from build123d import *

# Parameters (mm, degrees)
F1_W      = 2334
F1_H      = 613
F2_DEPTH  = 30
F3_W      = 45
F3_H      = 420
F3_W_2    = 982.5
F3_H_2    = 45
F4_DEPTH  = 70
F5_DEPTH  = 870
F8_W      = 45
F8_H      = 420
F9_DEPTH  = 70
F10_DEPTH = 670
F11_DEPTH = 70


# Not quite as in the source:
# - a feature names something its author has since deleted; it is built from what else it names


with BuildPart() as f2:
    # F1 (on offset) → F2 (new body)
    with BuildSketch(Plane.XY.offset(900)):
        Rectangle(F1_W, F1_H)
    extrude(amount=-F2_DEPTH)

    # F3 (on face) → F4 (join)
    with BuildSketch(Plane(origin=(0, 0, 870), x_dir=(1, 0, 0), z_dir=(0, 0, -1))):
        with Locations((-1102.5, 0)):
            Rectangle(F3_W, F3_H)
        with Locations((1102.5, 0)):
            Rectangle(F3_W, F3_H)
        with Locations((-538.75, 232.5)):
            Rectangle(F3_W_2, F3_H_2)
        with Locations((-538.75, -232.5)):
            Rectangle(F3_W_2, F3_H_2)
        Polygon((47.5, 255), (-47.5, 255), (-47.5, 210), (-22.5, 210), (22.5, 210), (47.5, 210), align=None)
        with Locations((538.75, 232.5)):
            Rectangle(F3_W_2, F3_H_2)
        Polygon((22.5, 210), (-22.5, 210), (-22.5, -210), (22.5, -210), (22.5, -47.5), (22.5, 47.5), align=None)
        with Locations((538.75, -232.5)):
            Rectangle(F3_W_2, F3_H_2)
    extrude(amount=F4_DEPTH)

    # F3 (on face) → F5 (join)
    with BuildSketch(Plane(origin=(0, 0, 870), x_dir=(1, 0, 0), z_dir=(0, 0, -1))):
        Polygon((-1030, 255), (-1125, 255), (-1125, 210), (-1080, 210), (-1030, 210), align=None)
        Polygon((47.5, 255), (-47.5, 255), (-47.5, 210), (-22.5, 210), (22.5, 210), (47.5, 210), align=None)
        Polygon((-1080, -210), (-1125, -210), (-1125, -255), (-1030, -255), (-1030, -210), align=None)
        Polygon((1125, 255), (1030, 255), (1030, 210), (1080, 210), (1125, 210), align=None)
        Polygon((22.5, -210), (-22.5, -210), (-47.5, -210), (-47.5, -255), (47.5, -255), (47.5, -210), align=None)
        Polygon((1125, -255), (1125, -210), (1080, -210), (1030, -210), (1030, -255), align=None)
    extrude(amount=F5_DEPTH)

    # F8 (on offset) → F9 (join)
    with BuildSketch(Plane.XY.offset(130)):
        Polygon((-638, 210), (-638, 255), (-1100, 255), (-1100, -255), (-638, -255), (-638, -210), (-1055, -210), (-1055, 210), align=None)
        Polygon((568, 210), (568, 255), (-568, 255), (-568, 210), (-22.5, 210), (22.5, 210), align=None)
        Polygon((-568, -255), (568, -255), (568, -210), (22.5, -210), (-22.5, -210), (-568, -210), align=None)
        Rectangle(F8_W, F8_H)
        Polygon((1100, -255), (1100, 255), (638, 255), (638, 210), (1055, 210), (1055, -210), (638, -210), (638, -255), align=None)
    extrude(amount=F9_DEPTH)

    # F8 (on offset) → F10 (join, through all)
    with BuildSketch(Plane.XY.offset(130)):
        Polygon((-638, -255), (-568, -255), (-568, -210), (-580.5, -210), (-625.5, -210), (-638, -210), align=None)
        Polygon((-568, 210), (-568, 255), (-638, 255), (-638, 210), (-625.5, 210), (-580.5, 210), align=None)
        Polygon((638, 210), (638, 255), (568, 255), (568, 210), (580.5, 210), (625.5, 210), align=None)
        Polygon((568, -255), (638, -255), (638, -210), (625.5, -210), (580.5, -210), (568, -210), align=None)
    extrude(amount=F10_DEPTH)

    # F8 (on offset) → F11 (join)
    with BuildSketch(Plane.XY.offset(130)):
        with Locations((-603, 0)):
            Rectangle(F8_W, F8_H)
        with Locations((603, 0)):
            Rectangle(F8_W, F8_H)
    extrude(amount=F11_DEPTH)


solid = f2.part
Could you check a few things on this model? Use its own coordinates, in mm. A direction names the side the tool comes from. Coordinates: 2 decimals unless noted, no trailing zeros. Write each loop counter-clockwise with the first axis right and the second up, starting at its lowest first coordinate (ties: lowest second). Pieces come first, ordered by that corner, then holes. Notation, with made-up numbers: (-38, -37.75) - (-10, -37.75) arc R15 cw to (-10, -16.75) - close; hole circle Ø3 at (27, -19). An arc over 180 degrees is marked (long way). Write item = value, one per line.
1) Suppose I cut it at B-B on z = 99. Please give me the cut outline in (x, y).
Result set:
outline = (-1125, -255) - (-1030, -255) - (-1030, -210) - (-1125, -210) - close; (-1125, 210) - (-1030, 210) - (-1030, 255) - (-1125, 255) - close; (-47.5, -255) - (47.5, -255) - (47.5, -210) - (-47.5, -210) - close; (-47.5, 210) - (47.5, 210) - (47.5, 255) - (-47.5, 255) - close; (1030, -255) - (1125, -255) - (1125, -210) - (1030, -210) - close; (1030, 210) - (1125, 210) - (1125, 255) - (1030, 255) - close
2) Suppose I cut it at A-A on x = -153.5. Please give me the cut outline in (y, z).
Result set:
outline = (-306.5, 870) - (-255, 870) - (-255, 800) - (-210, 800) - (-210, 870) - (210, 870) - (210, 800) - (255, 800) - (255, 870) - (306.5, 870) - (306.5, 900) - (-306.5, 900) - close; (-255, 130) - (-210, 130) - (-210, 200) - (-255, 200) - close; (210, 130) - (255, 130) - (255, 200) - (210, 200) - close
3) We'd pull the mould along Y, two halves only. Please class faces 1 (the flat face through (304, 232, 800)), 2 (the flat face through (580.5, -3, 165)): +Y half, -Y half, draft (parallel to the pull), parting line (faces both ways), or undercut.
Result set:
face_1 = draft
face_2 = undercut
4) Will these pins go through, and if not, where does the flat tip stop? pin 1 Ø3 at (x, y) = (652.5, -45.5) entering from -Z; pin 2 Ø21 at (y, z) = (55.5, 181.5) entering from -X; pin 3 Ø1 at (x, y) = (587.5, -33) entering from -Z.
Result set:
pin_1 = 870
pin_2 = -1100
pin_3 = 130
5) Please list where these lines run through material, in increasing order: line 1 (X direction, y = 246, z = 449); line 2 (X direction, y = 101, z = 192.5); line 3 (Y direction, x = 158.5, z = 173.5). Write a range as [from, to].
Result set:
line_1 = [-1125, -1030], [-638, -568], [-47.5, 47.5], [568, 638], [1030, 1125]
line_2 = [-1100, -1055], [-625.5, -580.5], [-22.5, 22.5], [580.5, 625.5], [1055, 1100]
line_3 = [-255, -210], [210, 255]
6) Suppose I cut it at C-C on y = 92.5. State how many separate pieces and enclosed holes the cut face has, plus the area to 3 significant figures.
Result set:
separate_pieces = 6
enclosed_holes = 0
area = 95,200 mm2
7) For faces 3 (the flat face through (831, -232, 200)), 4 (the flat face through (1100, -3, 165)), 5 (the flat face through (22.5, 3, 835)), which set-ups out of +Z, -Z, +X, -X, +Y, -Y let a thin tool reach every point of the face, with its end or its side?
Result set:
face_3 = +Y, -Y
face_4 = -Z, +X
face_5 = -Z
